Here's how the part is built. I have some questions about the finished solid (model axes, mm). A direction names the side the tool comes from. Round coordinates to 2 decimals unless told otherwise and drop trailing zeros. Order: outer loops, then holes, each group sorted by start corner. A loop starts at its lowest first (then second) coordinate and runs counter-clockwise, first axis right, second up. Notation, with made-up numbers: M 48,-24 L 69,-24 A25 ccw 69,11 Z; hole C 56,46 d11. An arc over 180 degrees is marked long. Write item = value, one per line. Start each with the question number.
Item 1: I want a section at C-C, the plane x = -6. List the corners of the cut face in (y, z) for me, plus the area to 3 significant figures.
Item 2: I'm going to push a flat-ended pin straight in: P1, Ø2, axis at y = 91.5, z = -17.5, coming from the +X side. Where does the tip first touch, or does it pass through?
Item 3: Please list where these lines run through material, in increasing order: L1, parallel to Y at x = -30, z = 21; L2, parallel to X at y = 42.5, z = 21; L3, parallel to Z at x = 19, y = 96.5.
Item 4: For faces 5 (the face through (14.836, 21.914, -28.132)), 6 (the face through (-21.85, 16.97, -12.2)), 7 (the face through (-27, 21.089, 5)), 8 (the face through (-20.945, 79, -1)), 9 (the face through (-26.984, 120.739, -32.92)), which set-ups out of +Z, -Z, +X, -X, +Y, -Y let a thin tool reach every point of the face, with its end or its side?
Item 5: I want a section at D-D, the plane y = 43. List the corners of the cut face in (x, z) for me, plus the area to 3 significant figures.
Item 6: We'd pull the mould along Y, two halves only. Please class faces 1 (the face through (-27, 108, 24.98)), 2 (the face through (-30, 114.3, -36)), 3 (the face through (-27.206, 85.455, -19.152)), 4 (the face through (-27, 27.439, 4)): pulls with the +Y half, pulls with the -Y half, needs draft (parallel to the pull), parting line crosses it, or undercut.
Item 7: I want a section at B-B, the plane y = 116.5. List the corners of the cut face in (x, z) for me (3 decimals).
Item 8: I want a section at A-A, the plane z = 9. List the corners of the cut face in (x, y) for me, plus the area to 3 significant figures.
```python
from build123d import *

# Parameters (mm, degrees)
F0_W     = 64.7085476667
F0_H     = 64.7085476667
F1_DEPTH = 127
F2_W     = 52.0085476667
F2_H     = 52.0085476667
F3_DEPTH = 127.001
F5_DEPTH = 44.45
F6_W     = 6.35
F6_H     = 24.2487721393
F7_DEPTH = 12.701
F9_DEPTH = 12.7


# Not quite as in the source:
# - a feature names something its author has since deleted; it is built from what else it names


with BuildPart() as f1:
    # F0 (on Front) → F1 (new body)
    with BuildSketch(Plane.XZ):
        with Locations((-1.2904843315, -7.374192588)):
            Rectangle(F0_W, F0_H)
    extrude(amount=-F1_DEPTH)

    # F2 (on face) → F3 (cut, through all)
    with BuildSketch(Plane(origin=(0, 127, 0), x_dir=(-1, 0, 0), z_dir=(0, 1, 0))):
        with Locations((-5.0595156685, -1.024192588)):
            Rectangle(F2_W, F2_H)
    extrude(amount=-F3_DEPTH, mode=Mode.SUBTRACT)

    # F4 (on face) → F5 (cut)
    with BuildSketch(Plane.XZ):
        Polygon((31.0637895018, -27.0284664214), (-0.9437288021, -27.0284664214), (31.0637895018, -29.2666501498), align=None)
        Polygon((-20.9447581649, -25.6298581929), (-20.9447581649, 0.731309106), (-22.7791408762, -25.5015856572), align=None)
    extrude(amount=-F5_DEPTH, mode=Mode.SUBTRACT)

    # F6 (on face) → F7 (cut, through all)
    with BuildSketch(Plane.YZ.offset(-20.9447581649)):
        with Locations((24.2636220248, 12.8556951756)):
            Rectangle(F6_W, F6_H)
        with BuildLine():
            Line((27.4386220248, -15.9778556544), (27.4386220248, 0.731309106))
            Line((27.4386220248, 0.731309106), (21.0886220248, 0.731309106))
            Line((21.0886220248, 0.731309106), (21.0886220248, -15.9778556544))
            ThreePointArc((21.0886220248, -15.9778556544), (24.2636220248, -19.1528556544), (27.4386220248, -15.9778556544))
        make_face()
        with BuildLine():
            Line((88.7001905876, 24.9800812453), (82.3501905876, 24.9800812453))
            Line((82.3501905876, 24.9800812453), (82.3501905876, -15.9781904151))
            ThreePointArc((82.3501905876, -15.9781904151), (85.5251905876, -19.1531904151), (88.7001905876, -15.9781904151))
            Line((88.7001905876, -15.9781904151), (88.7001905876, 24.9800812453))
        make_face()
    extrude(amount=-F7_DEPTH, mode=Mode.SUBTRACT)

    # F8 (on face) → F9 (cut)
    with BuildSketch(Plane(origin=(0, 127, 0), x_dir=(-1, 0, 0), z_dir=(0, 1, 0))):
        with BuildLine():
            Line((33.6447581649, -39.7284664214), (33.6447581649, -30.2034664214))
            ThreePointArc((33.6447581649, -30.2034664214), (26.9095660741, -32.9932743306), (24.1197581649, -39.7284664214))
            Line((24.1197581649, -39.7284664214), (33.6447581649, -39.7284664214))
        make_face()
    extrude(amount=-F9_DEPTH, mode=Mode.SUBTRACT)


solid = f1.part
```
Filled in:
q1.outline = M 0,-39.73 L 127,-39.73 L 127,-27.03 L 0,-27.03 Z
q1.area = 1,610 mm^2
q2.P1 = -20.94
q3.L1 = 0 to 21.09, 27.44 to 82.35, 88.7 to 127
q3.L2 = -33.64 to -20.94
q3.L3 = -39.73 to -27.03
q4.face_5 = +Z, +X, -Y
q4.face_6 = +X, -Y
q4.face_7 = +Z, +X, -X
q4.face_8 = +Z, +X, +Y, -Y
q4.face_9 = -Z, -X, +Y
q5.outline = M -33.64,-39.73 L 31.06,-39.73 L 31.06,-29.27 L -0.94,-27.03 L -20.94,-27.03 L -20.94,-25.63 L -22.78,-25.5 L -20.94,0.73 L -20.94,24.98 L -33.64,24.98 Z
q5.area = 1,420 mm^2
q6.face_1 = needs draft
q6.face_2 = pulls with the +Y half
q6.face_3 = undercut
q6.face_4 = undercut
q7.outline = M -33.645,-30.203 A9.525 cw -24.12,-39.728 L 31.064,-39.728 L 31.064,-27.028 L -20.945,-27.028 L -20.945,24.98 L -33.645,24.98 Z
q8.outline = M -33.64,0 L -20.94,0 L -20.94,21.09 L -33.64,21.09 Z; M -33.64,27.44 L -20.94,27.44 L -20.94,82.35 L -33.64,82.35 Z; M -33.64,88.7 L -20.94,88.7 L -20.94,127 L -33.64,127 Z
q8.area = 1,450 mm^2
